```python
from build123d import *

# Parameters (mm, degrees)
SKETCH1_R               = 25
SKETCH1_R_2             = 18.65
BOSS_EXTRUDE1_DEPTH     = 685.8
CUT_EXTRUDE1_DEPTH      = 687.710739686
CUT_EXTRUDE1_DEPTH_BACK = 687.710739686
SKETCH2_R               = 4.7625


with BuildPart() as part:
    # Sketch1 → Boss-Extrude1 (new body)
    with BuildSketch(Plane.XY):
        Circle(SKETCH1_R)
        Circle(SKETCH1_R_2, mode=Mode.SUBTRACT)
    extrude(amount=BOSS_EXTRUDE1_DEPTH)

    # Sketch2 → Cut-Extrude1 (cut, two sides: drawn at the far end of the back side and taken through both)
    with BuildSketch(Plane(origin=(0, 0, 0), x_dir=(0, 0, -1), z_dir=(1, 0, 0)).offset(-CUT_EXTRUDE1_DEPTH_BACK)):
        with Locations((-647.7, 0)):
            Circle(SKETCH2_R)
        with Locations((-38.1, 0)):
            Circle(SKETCH2_R)
    extrude(amount=CUT_EXTRUDE1_DEPTH + CUT_EXTRUDE1_DEPTH_BACK, mode=Mode.SUBTRACT)


solid = part.part
```
Model file for the job. Use its own axes, mm. Coordinates: 2 decimals unless noted, no trailing zeros. Write each loop counter-clockwise with the first axis right and the second up, starting at its lowest first coordinate (ties: lowest second). Pieces come first, ordered by that corner, then holes. Notation, with made-up numbers: (21, 22.5) - (75, 22.5) arc R29 cw to (75, 45.5) - close; hole circle Ø4 at (-6.75, -40). An arc over 180 degrees is marked (long way). Use a Markdown table: item, result. Add a question column.
Item 1: Band-saw the part on B-B, the plane y = -11. Write the cut outline in (x, z).
Item 2: Band-saw the part on C-C, the plane z = 220. Write the cut outline in (x, y), and give its area (3 significant figures).
Item 3: Band-saw the part on A-A, the plane x = 0. Write the cut outline in (y, z).
Item 4: Two-plate mould, pull along Y, no slides. Class faces 1 (the face through (-14.8, -11.35, 338.1)), 2 (the face through (23.846, 7.509, 338.099)), 3 (the face through (-19, -2, 685.8)): pulls with the +Y half, pulls with the -Y half, needs draft (parallel to the pull), parting line crosses it, or undercut.
Item 5: Drill centre lines: line 1 along Z through (x, y) = (23.25, 0); line 2 along X through (y, z) = (17, 544). Where is each one in solid material? Low to high.
Item 6: Drop flat-ended pins along their axis: pin 1 (4 mm diameter, centred on y = -18, z = 319, fed in from +X); pin 2 (5 mm diameter, centred on y = 3.5, z = 616, fed in from +X); pin 3 (7.5 mm diameter, centred on y = 0, z = 38.1, fed in from +X); pin 4 (10 mm diameter, centred on y = -17.5, z = 580, fed in from -X). Give the stop position or say it passes through.
A:
| question | item | result |
|---|---|---|
| 1 | outline | (-22.45, 0) - (-15.06, 0) - (-15.06, 685.8) - (-22.45, 685.8) - close; (15.06, 0) - (22.45, 0) - (22.45, 685.8) - (15.06, 685.8) - close |
| 2 | outline | circle Ø50 at (0, 0); hole circle Ø37.3 at (0, 0) |
| 2 | area | 871 mm² |
| 3 | outline | (-25, 0) - (-18.65, 0) - (-18.65, 685.8) - (-25, 685.8) - close; (18.65, 0) - (25, 0) - (25, 685.8) - (18.65, 685.8) - close |
| 4 | face 1 | undercut |
| 4 | face 2 | parting line crosses it |
| 4 | face 3 | needs draft |
| 5 | line 1 | z = 0 to 33.34, 42.86 to 642.94, 652.46 to 685.8 |
| 5 | line 2 | x = -18.33 to -7.67, 7.67 to 18.33 |
| 6 | pin 1 | stops at x = 19.21 |
| 6 | pin 2 | stops at x = 24.98 |
| 6 | pin 3 | passes through |
| 6 | pin 4 | stops at x = -21.65 |
